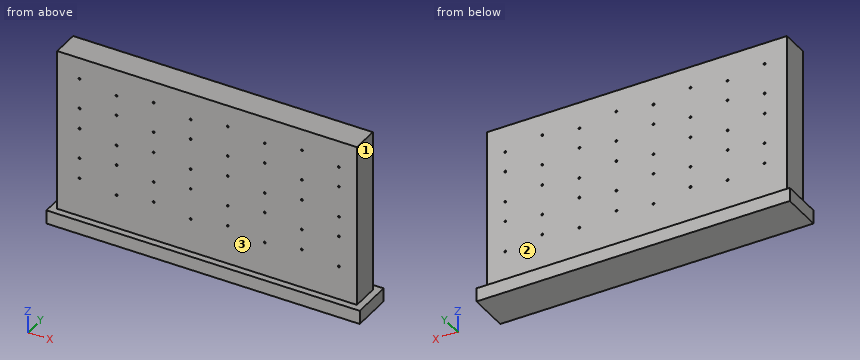
from build123d import *

# Parameters (mm, degrees)
SKETCH1_W           = 292.1
SKETCH1_H           = 38.1
BOSS_EXTRUDE1_DEPTH = 12.7
SKETCH2_W           = 279.4
SKETCH2_H           = 25.4
BOSS_EXTRUDE2_DEPTH = 152.4
SKETCH4_R           = 0.875
CUT_EXTRUDE1_DEPTH  = 223.703109543


with BuildPart() as part:
    # Sketch1 → Boss-Extrude1 (new body)
    with BuildSketch(Plane.XY):
        Rectangle(SKETCH1_W, SKETCH1_H)
    extrude(amount=BOSS_EXTRUDE1_DEPTH)

    # Sketch2 → Boss-Extrude2 (add)
    with BuildSketch(Plane.XY.offset(12.7)):
        Rectangle(SKETCH2_W, SKETCH2_H)
    extrude(amount=BOSS_EXTRUDE2_DEPTH)

    # Sketch4 → Cut-Extrude1 (cut, through all)
    with BuildSketch(Plane.XZ.offset(12.7)):
        with Locations(Location((-118.894764252, 116.542067709, 0), (0, 0, 270))):
            Circle(SKETCH4_R)
        with Locations(Location((-118.894764252, 68.536067709, 0), (0, 0, 270))):
            Circle(SKETCH4_R)
        with Locations(Location((-84.394764252, 73.351013878, 0), (0, 0, 270))):
            Circle(SKETCH4_R)
        with Locations(Location((-118.894764252, 49.10609229, 0), (0, 0, 270))):
            Circle(SKETCH4_R)
        with Locations(Location((-84.394764252, 44.291146122, 0), (0, 0, 270))):
            Circle(SKETCH4_R)
        with Locations(Location((-49.806764252, 68.536067709, 0), (0, 0, 270))):
            Circle(SKETCH4_R)
        with Locations(Location((-49.806764252, 116.542067709, 0), (0, 0, 270))):
            Circle(SKETCH4_R)
        with Locations(Location((-49.806764252, 145.10793229, 0), (0, 0, 270))):
            Circle(SKETCH4_R)
        with Locations(Location((-15.306764252, 44.291146122, 0), (0, 0, 270))):
            Circle(SKETCH4_R)
        with Locations(Location((-15.306764252, 73.351013878, 0), (0, 0, 270))):
            Circle(SKETCH4_R)
        with Locations(Location((19.281235748, 116.542067709, 0), (0, 0, 270))):
            Circle(SKETCH4_R)
        with Locations(Location((19.281235748, 145.10793229, 0), (0, 0, 270))):
            Circle(SKETCH4_R)
        with Locations(Location((53.781235748, 121.357013878, 0), (0, 0, 270))):
            Circle(SKETCH4_R)
        with Locations(Location((122.869235748, 92.292066122, 0), (0, 0, 270))):
            Circle(SKETCH4_R)
        with Locations(Location((88.369235748, 68.536067709, 0), (0, 0, 270))):
            Circle(SKETCH4_R)
        with Locations(Location((88.369235748, 49.10609229, 0), (0, 0, 270))):
            Circle(SKETCH4_R)
        with Locations(Location((122.869235748, 44.291146122, 0), (0, 0, 270))):
            Circle(SKETCH4_R)
        with Locations(Location((122.869235748, 73.351013878, 0), (0, 0, 270))):
            Circle(SKETCH4_R)
        with Locations(Location((88.369235748, 97.10701229, 0), (0, 0, 270))):
            Circle(SKETCH4_R)
        with Locations(Location((-118.894764252, 145.10793229, 0), (0, 0, 270))):
            Circle(SKETCH4_R)
        with Locations(Location((-84.394764252, 140.292986122, 0), (0, 0, 270))):
            Circle(SKETCH4_R)
        with Locations(Location((-84.394764252, 121.357013878, 0), (0, 0, 270))):
            Circle(SKETCH4_R)
        with Locations(Location((-118.894764252, 97.10701229, 0), (0, 0, 270))):
            Circle(SKETCH4_R)
        with Locations(Location((-84.394764252, 92.292066122, 0), (0, 0, 270))):
            Circle(SKETCH4_R)
        with Locations(Location((-49.806764252, 49.10609229, 0), (0, 0, 270))):
            Circle(SKETCH4_R)
        with Locations(Location((-49.806764252, 97.10701229, 0), (0, 0, 270))):
            Circle(SKETCH4_R)
        with Locations(Location((-15.306764252, 140.292986122, 0), (0, 0, 270))):
            Circle(SKETCH4_R)
        with Locations(Location((-15.306764252, 92.292066122, 0), (0, 0, 270))):
            Circle(SKETCH4_R)
        with Locations(Location((19.281235748, 49.10609229, 0), (0, 0, 270))):
            Circle(SKETCH4_R)
        with Locations(Location((19.281235748, 68.536067709, 0), (0, 0, 270))):
            Circle(SKETCH4_R)
        with Locations(Location((19.281235748, 97.10701229, 0), (0, 0, 270))):
            Circle(SKETCH4_R)
        with Locations(Location((53.781235748, 140.292986122, 0), (0, 0, 270))):
            Circle(SKETCH4_R)
        with Locations(Location((88.369235748, 145.10793229, 0), (0, 0, 270))):
            Circle(SKETCH4_R)
        with Locations(Location((122.869235748, 140.292986122, 0), (0, 0, 270))):
            Circle(SKETCH4_R)
        with Locations(Location((122.869235748, 121.357013878, 0), (0, 0, 270))):
            Circle(SKETCH4_R)
        with Locations(Location((88.369235748, 116.542067709, 0), (0, 0, 270))):
            Circle(SKETCH4_R)
        with Locations(Location((53.781235748, 44.291146122, 0), (0, 0, 270))):
            Circle(SKETCH4_R)
        with Locations(Location((53.781235748, 92.292066122, 0), (0, 0, 270))):
            Circle(SKETCH4_R)
        with Locations(Location((53.781235748, 73.351013878, 0), (0, 0, 270))):
            Circle(SKETCH4_R)
        with Locations(Location((-15.306764252, 121.357013878, 0), (0, 0, 270))):
            Circle(SKETCH4_R)
    extrude(amount=-CUT_EXTRUDE1_DEPTH, mode=Mode.SUBTRACT)


solid = part.part
For this review, take the finished solid that the model builds, in its own axes (mm). Face numbers are marked on the shaded views. A direction names the side the tool comes from. Give positions to 0.01 mm unless a question says otherwise; leave off trailing zeros. Loops run counter-clockwise (first coordinate to the right, second up) from the corner with the lowest first, then second, coordinate; pieces in that order, holes last.
Item 1: Take a section at B-B, the plane z = 133. State the section outline as (x, y) points, and give its area (3 significant figures).
Item 2: For line 1 along X through (y, z) = (0, 91.5); line 2 along Z through (x, y) = (35, -14); line 3 along X through (y, z) = (-5, 118.5), list the stretches that pass through material, from the lowest coordinate up.
Item 3: Take a section at C-C, the plane y = -0.5. Give the number of separate pieces and of enclosed holes in the cut face, and give its area (3 significant figures).
Item 4: Insertion check: pin 1 (1 mm diameter, centred on x = 39, z = 91, fed in from +Y); pin 2 (1.4 mm diameter, centred on x = -118.89, z = 49.11, fed in from +Y); pin 3 (2.5 mm diameter, centred on x = 19.28, z = 49.11, fed in from -Y); pin 4 (10 mm diameter, centred on y = 12.5, z = 104.5, fed in from -X). Each pin has a flat end and moves straight along its axis. Give the tip position at first contact, or say it passes through.
Item 5: Take a section at A-A, the plane x = -99. State the section outline as (y, z) points, and give its area (3 significant figures).
Item 6: Tool access review of the marked faces 1, 2 and 3: name each direction out of +Z, -Z, +X, -X, +Y, -Y from which nothing blocks a thin tool from reaching the whole face with its end or side.
Calculated:
1. outline: (-139.7, -12.7) - (139.7, -12.7) - (139.7, 12.7) - (-139.7, 12.7) - close
1. area: 7,100 mm2
2. line 1: x = -139.7 to -84.77, -84.02 to -15.68, -14.93 to 53.41, 54.15 to 122.5, 123.24 to 139.7
2. line 2: z = 0 to 12.7
2. line 3: x = -139.7 to 139.7
3. separate pieces: 1
3. enclosed holes: 40
3. area: 46,200 mm2
4. pin 1: stops at y = 12.7
4. pin 2: passes through
4. pin 3: stops at y = -12.7
4. pin 4: stops at x = -139.7
5. outline: (-19.05, 0) - (19.05, 0) - (19.05, 12.7) - (12.7, 12.7) - (12.7, 165.1) - (-12.7, 165.1) - (-12.7, 12.7) - (-19.05, 12.7) - close
5. area: 4,350 mm2
6. face 1: +Z, +X, +Y, -Y
6. face 2: +Z, +X, -X, +Y
6. face 3: +Z, +X, -X, -Y
